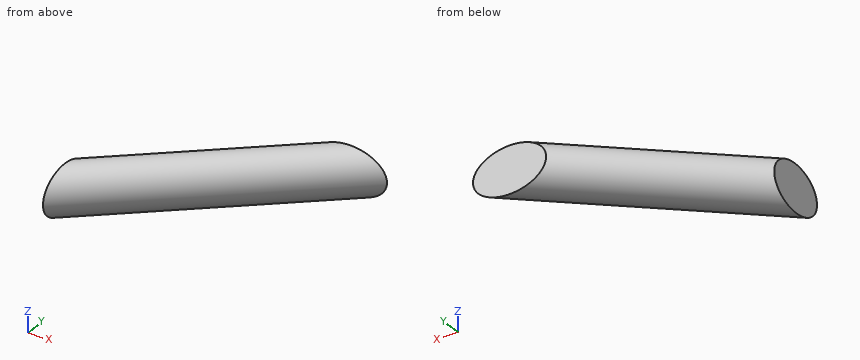
from build123d import *

# Parameters (mm, degrees)
CUT_EXTRUDE1_DEPTH      = 206.849628346
CUT_EXTRUDE1_DEPTH_BACK = 206.849628346
CUT_EXTRUDE2_DEPTH      = 185.85731066
CUT_EXTRUDE2_DEPTH_BACK = 185.85731066


with BuildPart() as part:
    # Sketch1 → Revolve-Thin1 (revolve)
    with BuildSketch(Plane.XY, mode=Mode.PRIVATE) as revolve_thin1_sk:
        Polygon((135.605846103, 117.01106453), (-94.788032894, -82.542688932), (-78.158553439, -101.742178848), (152.235325558, 97.811574614), align=None)
    revolve(revolve_thin1_sk.sketch.rotate(Axis((135.605846103, 117.01106453, 0), (-0.7558854297800033, -0.6547039155574831, 0)), 180), axis=Axis((135.605846103, 117.01106453, 0), (-0.7558854297800033, -0.6547039155574831, 0)))

    # Sketch2 → Cut-Extrude1 (cut, two sides: drawn at the far end of the back side and taken through both)
    with BuildSketch(Plane.XY.offset(-CUT_EXTRUDE1_DEPTH_BACK)):
        Polygon((180.039707564, 97.811574614), (7.480130989, 97.811574614), (101.41164362, 186.9937411), align=None)
    extrude(amount=CUT_EXTRUDE1_DEPTH + CUT_EXTRUDE1_DEPTH_BACK, mode=Mode.SUBTRACT)

    # Sketch3 → Cut-Extrude2 (cut, two sides: drawn at the far end of the back side and taken through both)
    with BuildSketch(Plane.XY.offset(-CUT_EXTRUDE2_DEPTH_BACK)):
        Polygon((-78.158553439, -101.742178848), (-78.158553439, 0), (-164.424224952, -9.260462321), (-121.291389196, -114.506813698), align=None)
    extrude(amount=CUT_EXTRUDE2_DEPTH + CUT_EXTRUDE2_DEPTH_BACK, mode=Mode.SUBTRACT)


solid = part.part
Can you work these out from the model? Positions are in its coordinate system, mm. Give positions to 0.01 mm unless a question says otherwise; leave off trailing zeros. Loops run counter-clockwise (first coordinate to the right, second up) from the corner with the lowest first, then second, coordinate; pieces in that order, holes last. Notation, with made-up numbers: M -31,36 L -17,36 A32 ccw -17,67 Z; hole C 81.5,19.5 d4. An arc over 180 degrees is marked long. One line per item, written item: value.
1) I'm going to push flat-ended pins straight in: pin 1 (1.5 mm diameter, centred on y = 62, z = 12, fed in from +X); pin 2 (5 mm diameter, centred on x = -26, z = -11.5, fed in from -Y); pin 3 (3 mm diameter, centred on y = 55.5, z = -13, fed in from -X); pin 4 (2 mm diameter, centred on x = -12, y = 26, fed in from -Z). Where does each tip first touch, or does it pass through?
Geometry check:
pin 1: stops at x = 107.34
pin 2: stops at y = -55.59
pin 3: stops at x = 29.09
pin 4: passes through
2) Please list where these lines run through material, in increasing order: line 1 (Y direction, x = 130, z = 12); line 2 (Y direction, x = 45.5, z = -17.5); line 3 (X direction, y = 74, z = 12.5).
Geometry check:
line 1: y = 82.54 to 97.81
line 2: y = 14.61 to 63.32
line 3: x = 52.17 to 119.72
3) Imagine slicing it at A-A on z = -9.5. Write out the boundary of the cut face in (x, y).
Geometry check:
outline: M -78.16,-99.3 L 149.42,97.81 L 77.46,97.81 L -78.16,-36.98 Z
